For this review, take the finished solid that the model builds, in its own axes (mm). Face numbers are marked on the shaded views. Coordinates: 2 decimals unless noted, no trailing zeros. Loops run counter-clockwise (first coordinate to the right, second up) from the corner with the lowest first, then second, coordinate; pieces in that order, holes last. Notation, with made-up numbers: (46.5, 75.25) - (51.5, 75.25) arc R18 cw to (51.5, 90.25) - close; hole circle Ø6 at (87.25, -36). An arc over 180 degrees is marked (long way). One line per item, written item: value. Start each with the question number.
1. Take a section at A-A, the plane x = -43.5. State the section outline as (y, z) points.
2. Insertion check: pin 1 (2.5 mm diameter, centred on x = 35.5, z = -19, fed in from +Y); pin 2 (6 mm diameter, centred on x = -36, z = -18.5, fed in from +Y); pin 3 (1.1 mm diameter, centred on x = 43, z = 7, fed in from +Y). Each pin has a flat end and moves straight along its axis. Give the tip position at first contact, or say it passes through.
3. Take a section at B-B, the plane z = 2. State the section outline as (x, y) points.
4. Take a section at D-D, the plane z = -19. State the section outline as (x, y) points, and give its area (3 significant figures).
5. To check wall thickness, follow line 1 (Z direction, x = -34.5, y = 4.65); line 2 (X direction, y = 3, z = 4.5); line 3 (Z direction, x = 5, y = 4). State the ranges of each line that lie inside material, in increasing order. Write a range as from..to.
6. The part is to be moulded in two halves that separate along Z. For the marked faces 1, 2 and 3, say which applies: released by +Z, released by -Z, zero draft, split by the parting line, or undercut.
```python
from build123d import *

# Parameters (mm, degrees)
SKETCH1_W           = 166.7
SKETCH1_H           = 70
BOSS_EXTRUDE2_DEPTH = 5
SKETCH2_W           = 69
SKETCH2_H           = 54
CUT_EXTRUDE1_DEPTH  = 3.5
SKETCH4_W           = 8.2
SKETCH4_H           = 20.89
CUT_EXTRUDE3_DEPTH  = 1.7
SKETCH3_W           = 17.75
SKETCH3_H           = 54
CUT_EXTRUDE4_DEPTH  = 2.4
SKETCH5_W           = 152.7
SKETCH5_H           = 2.3
CUT_EXTRUDE5_DEPTH  = 2.3
SKETCH6_W           = 37
SKETCH6_H           = 2.3
CUT_EXTRUDE7_DEPTH  = 2


with BuildPart() as part:
    # Sketch1 → Boss-Extrude2 (new body)
    with BuildSketch(Plane(origin=(0, 0, 0), x_dir=(1, 0, 0), z_dir=(0, 1, 0))):
        Rectangle(SKETCH1_W, SKETCH1_H)
    extrude(amount=BOSS_EXTRUDE2_DEPTH)

    # Sketch2 → Cut-Extrude1 (cut)
    with BuildSketch(Plane(origin=(0, 5, 0), x_dir=(1, 0, 0), z_dir=(0, 1, 0))):
        with Locations((-41.85, 1)):
            Rectangle(SKETCH2_W, SKETCH2_H)
    extrude(amount=-CUT_EXTRUDE1_DEPTH, mode=Mode.SUBTRACT)

    # Sketch4 → Cut-Extrude3 (cut)
    with BuildSketch(Plane(origin=(0, 5, 0), x_dir=(1, 0, 0), z_dir=(0, 1, 0))):
        with Locations((34.75, 15.555)):
            Rectangle(SKETCH4_W, SKETCH4_H)
        with Locations((47.95, 15.559824889)):
            Rectangle(SKETCH4_W, SKETCH4_H)
    extrude(amount=-CUT_EXTRUDE3_DEPTH, mode=Mode.SUBTRACT)

    # Sketch3 → Cut-Extrude4 (cut)
    with BuildSketch(Plane(origin=(0, 5, 0), x_dir=(1, 0, 0), z_dir=(0, 1, 0))):
        with Locations((67.475, 1)):
            Rectangle(SKETCH3_W, SKETCH3_H)
    extrude(amount=-CUT_EXTRUDE4_DEPTH, mode=Mode.SUBTRACT)

    # Sketch5 → Cut-Extrude5 (cut)
    with BuildSketch(Plane(origin=(0, 5, 0), x_dir=(1, 0, 0), z_dir=(0, 1, 0))):
        with Locations((0, -29.65)):
            Rectangle(SKETCH5_W, SKETCH5_H)
        with Locations((0, 31.65)):
            Rectangle(SKETCH5_W, SKETCH5_H)
    extrude(amount=-CUT_EXTRUDE5_DEPTH, mode=Mode.SUBTRACT)

    # Sketch6 → Cut-Extrude7 (cut)
    with BuildSketch(Plane(origin=(0, 5, 0), x_dir=(1, 0, 0), z_dir=(0, 1, 0))):
        with Locations((38.977751303, -19.59833207)):
            Rectangle(SKETCH6_W, SKETCH6_H)
        with Locations((38.977751303, -15.29833207)):
            Rectangle(SKETCH6_W, SKETCH6_H)
        with Locations((38.977751303, -10.99833207)):
            Rectangle(SKETCH6_W, SKETCH6_H)
        with Locations((38.977751303, -6.69833207)):
            Rectangle(SKETCH6_W, SKETCH6_H)
        with Locations((38.977751303, -23.89833207)):
            Rectangle(SKETCH6_W, SKETCH6_H)
    extrude(amount=-CUT_EXTRUDE7_DEPTH, mode=Mode.SUBTRACT)


solid = part.part
```
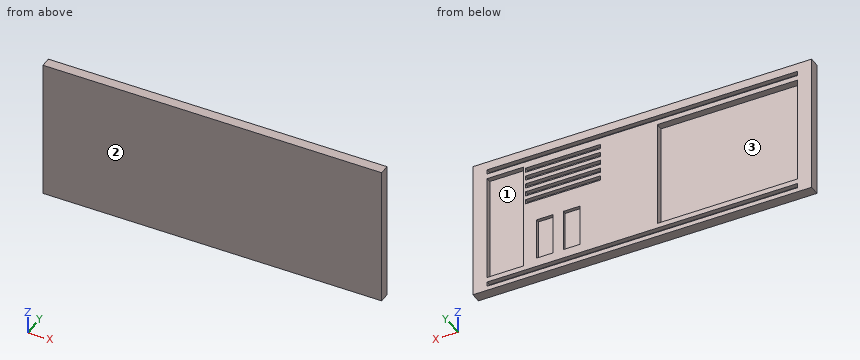
Solutions:
1. outline: (0, -35) - (5, -35) - (5, -32.8) - (2.7, -32.8) - (2.7, -30.5) - (5, -30.5) - (5, -28) - (1.5, -28) - (1.5, 26) - (5, 26) - (5, 28.5) - (2.7, 28.5) - (2.7, 30.8) - (5, 30.8) - (5, 35) - (0, 35) - close
2. pin 1: y = 3.3
2. pin 2: y = 1.5
2. pin 3: y = 3
3. outline: (-83.35, 0) - (83.35, 0) - (83.35, 5) - (76.35, 5) - (76.35, 2.6) - (58.6, 2.6) - (58.6, 5) - (-7.35, 5) - (-7.35, 1.5) - (-76.35, 1.5) - (-76.35, 5) - (-83.35, 5) - close
4. outline: (-83.35, 0) - (83.35, 0) - (83.35, 5) - (76.35, 5) - (76.35, 2.6) - (58.6, 2.6) - (58.6, 5) - (52.05, 5) - (52.05, 3.3) - (43.85, 3.3) - (43.85, 5) - (38.85, 5) - (38.85, 3.3) - (30.65, 3.3) - (30.65, 5) - (-7.35, 5) - (-7.35, 1.5) - (-76.35, 1.5) - (-76.35, 5) - (-83.35, 5) - close
4. area: 522 mm2
5. line 1: -35..-32.8, -30.5..-28, 26..28.5, 30.8..35
5. line 2: -83.35..-76.35, -7.35..58.6, 76.35..83.35
5. line 3: -35..-32.8, -30.5..28.5, 30.8..35
6. face 1: undercut
6. face 2: zero draft
6. face 3: undercut
